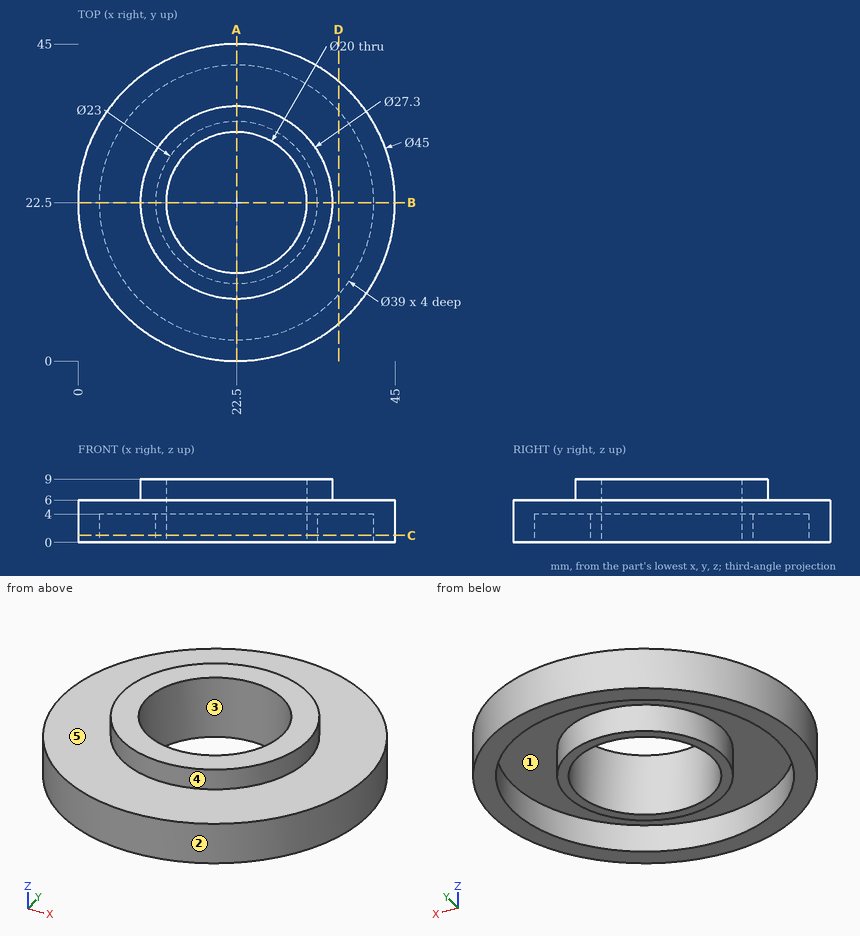
Study the drawing (mm; zero at the part's minimum x, y, z) and answer. A direction names the side the tool comes from. Give positions to 0.01 mm unless a question says otherwise; leave off trailing zeros. Write each loop counter-clockwise with the first axis right and the second up, starting at its lowest first coordinate (ties: lowest second). Pieces come first, ordered by that corner, then holes. Notation, with made-up numbers: (11.25, 22.5) -> (29.25, 22.5) arc R25 ccw to (29.25, 37.5) -> close; hole circle Ø3 at (-31.5, 80). An arc over 180 degrees is marked (long way). Answer as a JSON object with one key per item and string values. Group by question number.
1) Consider L1, parallel to Y at x = 22.5, z = 2.5; L2, parallel to Y at x = 31.5, z = 1.5; L3, parallel to X at y = 19.5, z = 1.75. Determine where each line is inside the solid, lowest interval first. Write a range as from..to.
2) The mould has two halves that part along X. Classify the marked faces 3, 4 and 5: +X half, -X half, draft (parallel to the pull), parting line (faces both ways), or undercut.
3) Find section D-D (x = 37). Write down the section's boundary in (y, z), and give its area (3 significant figures).
4) Find section C-C (z = 1). Write down the section's boundary in (x, y), and give its area (3 significant figures).
5) Find section A-A (x = 22.5). Write down the section's boundary in (y, z).
6) Each of these flat-tipped pins is pushed along its axis until it touches: P1, Ø4, axis at x = 10, z = 7, coming from the +Y side; P2, Ø5, axis at y = 30.5, z = 2, coming from the +X side; P3, Ø1.5, axis at x = 21.5, z = 2, coming from the +Y side. Where does it stop, or does it pass through?
7) A tool of negligible diameter and unlimited length cuts with its end or side. For the marked faces 1 and 2, from which of +Z, -Z, +X, -X, +Y, -Y can it reach the whole face along a straight path? Write none if from no direction.
Values follow:
{
 "1": {"L1": "y = 0..3, 11..12.5, 32.5..34, 42..45", "L2": "y = 1.88..5.2, 15.34..18.14, 26.86..29.66, 39.8..43.12", "L3": "x = 0.2..3.23, 11.4..12.96, 32.04..33.6, 41.77..44.8"},
 "2": {"face 3": "undercut", "face 4": "parting line", "face 5": "draft"},
 "3": {"outline": "(5.3, 0) -> (9.46, 0) -> (9.46, 4) -> (35.54, 4) -> (35.54, 0) -> (39.7, 0) -> (39.7, 6) -> (5.3, 6) -> close", "area": "102 mm2"},
 "4": {"outline": "circle Ø45 at (22.5, 22.5); circle Ø23 at (22.5, 22.5); hole circle Ø39 at (22.5, 22.5); hole circle Ø20 at (22.5, 22.5)", "area": "497 mm2"},
 "5": {"outline": "(0, 0) -> (3, 0) -> (3, 4) -> (11, 4) -> (11, 0) -> (12.5, 0) -> (12.5, 9) -> (8.85, 9) -> (8.85, 6) -> (0, 6) -> close; (32.5, 0) -> (34, 0) -> (34, 4) -> (42, 4) -> (42, 0) -> (45, 0) -> (45, 6) -> (36.15, 6) -> (36.15, 9) -> (32.5, 9) -> close"},
 "6": {"P1": "stops at y = 42.26", "P2": "stops at x = 44.32", "P3": "stops at y = 45"},
 "7": {"face 1": "-Z", "face 2": "+Z, -Z"}
}
